from build123d import *

# Parameters (mm, degrees)
SKETCH1_R               = 2.2500000000000004
BOSS_EXTRUDE1_DEPTH     = 14
BOSS_EXTRUDE2_DEPTH     = 30
SKETCH3_R               = 7
CUT_EXTRUDE1_DEPTH      = 15
FILLET1_R               = 5
RIB1_REACH              = 65.484
SKETCH4_WALL_W          = 136.0395678423848
SKETCH4_WALL_H          = 4
FILLET2_R               = 5
BOSS_EXTRUDE3_START     = -6
SKETCH6_W               = 50
SKETCH6_H               = 20.33166445293904
BOSS_EXTRUDE3_DEPTH     = 5
CUT_EXTRUDE2_REACH      = 73.338
SKETCH7_R               = 8.250000000000005
SKETCH7_R_2             = 8.25
FILLET3_R               = 5
FILLET4_R               = 5
RIB2_REACH              = 68.324
SKETCH8_WALL_W          = 155.84718590256796
SKETCH8_WALL_H          = 4
FILLET5_R               = 3
CUT_EXTRUDE3_DEPTH      = 20
FILLET6_R               = 2
CUT_EXTRUDE4_REACH      = 93.033
CUT_EXTRUDE4_END_RADIUS = 7
SKETCH10_R              = 3.5000000000000004


with BuildPart() as part:
    # Sketch1 → Boss-Extrude1 (new body)
    with BuildSketch(Plane.XY):
        with BuildLine():
            Line((9.2e-16, 7.5), (-14.999999999999998, 7.500000000000002))
            Line((-14.999999999999998, 7.500000000000002), (-14.999999999999998, -7.500000000000002))
            Line((-14.999999999999998, -7.500000000000002), (9.2e-16, -7.5))
            ThreePointArc((9.2e-16, -7.5), (7.5, 0), (9.2e-16, 7.5))
        make_face()
        Circle(SKETCH1_R, mode=Mode.SUBTRACT)
    extrude(amount=BOSS_EXTRUDE1_DEPTH)

    # Sketch2 → Boss-Extrude2 (add)
    with BuildSketch(Plane.ZY.offset(14.999999999999998)):
        Polygon((-28.999999999999993, -7.500000000000002), (43, -7.500000000000002), (42.99999999999999, 12.499999999999998), (-28.99999999999999, 12.499999999999998), align=None)
    extrude(amount=BOSS_EXTRUDE2_DEPTH)

    # Sketch3 → Cut-Extrude1 (cut)
    with BuildSketch(Plane.ZY.offset(45)):
        with Locations((28.999999999999996, 2.499999999999998)):
            Circle(SKETCH3_R)
        with Locations((-15, 2.499999999999998)):
            Circle(SKETCH3_R)
    extrude(amount=-CUT_EXTRUDE1_DEPTH, mode=Mode.SUBTRACT)

    # Fillet1
    fillet1_edges = [part.edges().sort_by_distance(p)[0] for p in [
        (-30, 12.499999999999998, -28.99999999999999),
        (-30, -7.500000000000002, -28.999999999999993),
        (-30, -7.500000000000002, 43),
        (-30, 12.499999999999998, 42.99999999999999),
    ]]
    fillet(fillet1_edges, radius=FILLET1_R)

    # Sketch4 wall → Rib1 (add, up to next)
    with BuildSketch(Plane(origin=(-12.5, 10, 14), x_dir=(0.707106781187, -0.707106781187, 0), z_dir=(0.707106781187, 0.707106781187, 0)), mode=Mode.PRIVATE) as rib1_sk1:
        with Locations((0, 2)):
            Rectangle(SKETCH4_WALL_W, SKETCH4_WALL_H)
    rib1_tool1 = extrude(rib1_sk1.sketch, amount=-RIB1_REACH, mode=Mode.PRIVATE) - part.part
    rib1 = rib1_tool1.solids().sort_by_distance((-12.5, 10, 14))[0]
    add(rib1)

    # Mirror1: Rib1 across plane
    add(rib1.mirror(Plane.XY.offset(7)))

    # Fillet2
    fillet2_edges = [part.edges().sort_by_distance(p)[0] for p in [
        (-10.000000000000002, 7.500000000000001, 2),
        (-10.000000000000002, 7.500000000000001, 12),
    ]]
    fillet(fillet2_edges, radius=FILLET2_R)

    # Sketch6 → Boss-Extrude3 (add)
    with BuildSketch(Plane.ZY.offset(45).offset(BOSS_EXTRUDE3_START)):
        with Locations((7.000000000000005, 22.665832226469526)):
            Rectangle(SKETCH6_W, SKETCH6_H)
    extrude(amount=-BOSS_EXTRUDE3_DEPTH)

    # Sketch7 → Cut-Extrude2 (cut, up to next)
    with BuildSketch(Plane.ZY.offset(39), mode=Mode.PRIVATE) as cut_extrude2_sk1:
        with Locations((-5.999999999999993, 22.665832226469526)):
            Circle(SKETCH7_R)
    cut_extrude2_tool1 = extrude(cut_extrude2_sk1.sketch, amount=-CUT_EXTRUDE2_REACH, mode=Mode.PRIVATE) & part.part
    # Sketch7 → Cut-Extrude2 (cut, up to next)
    with BuildSketch(Plane.ZY.offset(39), mode=Mode.PRIVATE) as cut_extrude2_sk2:
        with Locations((20.000000000000007, 22.665832226469526)):
            Circle(SKETCH7_R_2)
    cut_extrude2_tool2 = extrude(cut_extrude2_sk2.sketch, amount=-CUT_EXTRUDE2_REACH, mode=Mode.PRIVATE) & part.part
    add(cut_extrude2_tool1.solids().sort_by_distance((-39, 22.665832, -6))[0], mode=Mode.SUBTRACT)
    add(cut_extrude2_tool2.solids().sort_by_distance((-39, 22.665832, 20))[0], mode=Mode.SUBTRACT)

    # Fillet3
    fillet3_edges = [part.edges().sort_by_distance(p)[0] for p in [
        (-36.5, 12.500000000000004, -17.999999999999996),
        (-36.5, 12.500000000000004, 32.00000000000001),
    ]]
    fillet(fillet3_edges, radius=FILLET3_R)

    # Fillet4
    fillet4_edges = [part.edges().sort_by_distance(p)[0] for p in [
        (-36.5, 32.831664452939044, -17.999999999999996),
        (-36.5, 32.831664452939044, 32.00000000000001),
    ]]
    fillet(fillet4_edges, radius=FILLET4_R)

    # Sketch8 wall → Rib2 (add, up to next)
    with BuildSketch(Plane(origin=(-42, 22.665832227, 7), x_dir=(-0.283038838463, -0.959108448467, 0), z_dir=(0.959108448467, -0.283038838463, 0)), mode=Mode.PRIVATE) as rib2_sk1:
        Rectangle(SKETCH8_WALL_W, SKETCH8_WALL_H)
    rib2_tool1 = extrude(rib2_sk1.sketch, amount=RIB2_REACH, mode=Mode.PRIVATE) - part.part
    add(rib2_tool1.solids().sort_by_distance((-42, 22.665832227, 7))[0])

    # Fillet5
    fillet5_edges = [part.edges().sort_by_distance(p)[0] for p in [
        (-42, 12.5, 9),
        (-42, 12.5, 5),
    ]]
    fillet(fillet5_edges, radius=FILLET5_R)

    # Sketch9 → Cut-Extrude3 (cut)
    with BuildSketch(Plane.ZY.offset(45)):
        with BuildLine():
            Line((-10.499999999999998, 10.499999999999998), (24.500000000000004, 10.499999999999998))
            ThreePointArc((24.500000000000004, 10.499999999999998), (16.500000000000004, 2.4999999999999996), (24.500000000000004, -5.500000000000002))
            Line((24.500000000000004, -5.500000000000002), (-10.499999999999998, -5.500000000000002))
            ThreePointArc((-10.499999999999998, -5.500000000000002), (-2.4999999999999982, 2.4999999999999987), (-10.499999999999998, 10.499999999999998))
        make_face()
    extrude(amount=-CUT_EXTRUDE3_DEPTH, mode=Mode.SUBTRACT)

    # Fillet6
    fillet6_edges = [part.edges().sort_by_distance(p)[0] for p in [
        (-35, -5.500000000000002, -10.499999999999998),
        (-35, 10.5, -10.499999999999996),
        (-35, 10.499999999999998, 24.500000000000004),
        (-35, -5.500000000000002, 24.500000000000004),
    ]]
    fillet(fillet6_edges, radius=FILLET6_R - 0.0001)  # a hair under: the kernel refuses the full size

    # Cut-Extrude4: up to this cylinder (the profile starts outside it)
    cut_extrude4_end = Plane(origin=(-37.5, 2.499999999999998, -15), z_dir=(-1, 0, 0)) * Cylinder(CUT_EXTRUDE4_END_RADIUS, 201.066, mode=Mode.PRIVATE)
    # Sketch10 → Cut-Extrude4 (cut, up to the surface)
    with BuildSketch(Plane(origin=(0, 5.03e-15, -28.999999999999993), x_dir=(-1, 0, 0), z_dir=(0, 1.7e-16, -1)), mode=Mode.PRIVATE) as cut_extrude4_sk1:
        with Locations(Location((37.5, 2.499999999999993, 0), (0, 0, 90))):
            Circle(SKETCH10_R)
    cut_extrude4_tool1 = extrude(cut_extrude4_sk1.sketch, amount=-CUT_EXTRUDE4_REACH, mode=Mode.PRIVATE) - cut_extrude4_end
    cut_extrude4 = cut_extrude4_tool1.solids().sort_by_distance((-37.5, 2.5, -29))[0]
    add(cut_extrude4, mode=Mode.SUBTRACT)

    # Mirror2: Cut-Extrude4 across plane
    add(cut_extrude4.mirror(Plane.XY.offset(7)), mode=Mode.SUBTRACT)


solid = part.part
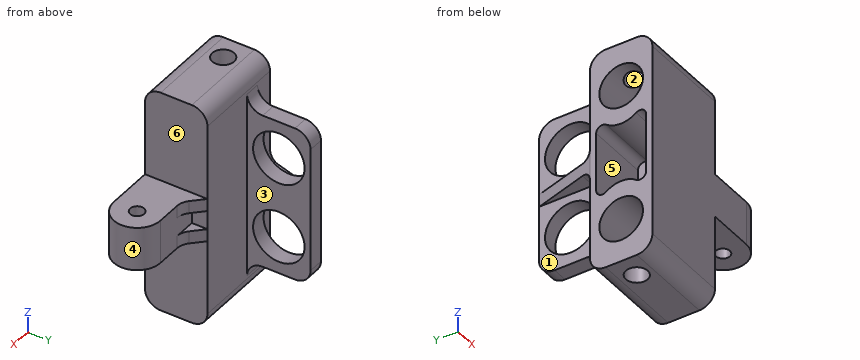
The listing builds one solid part. Answer for the finished solid, in the listing's coordinates (mm). Face numbers are marked on the shaded views. A direction names the side the tool comes from. Coordinates: 2 decimals unless noted, no trailing zeros. Order: outer loops, then holes, each group sorted by start corner. A loop starts at its lowest first (then second) coordinate and runs counter-clockwise, first axis right, second up.
Q1. A cutting plane is placed at B-B, the plane z = 7. Write down the section's boundary in (x, y), and give its area (3 significant figures).
Q2. For a pull along Y with two mould halves and no side action, classify the marked faces 4, 5 and 6 as pulls with the +Y half, pulls with the -Y half, needs draft (parallel to the pull), parting line crosses it, or undercut.
Q3. A cutting plane is placed at C-C, the plane y = 29.5. Write down the section's boundary in (x, z), and give its area (3 significant figures).
Q4. A cutting plane is placed at A-A, the plane z = -6. Write down the section's boundary in (x, y).
Q5. A cutting plane is placed at D-D, the plane z = -20. Write down the section's boundary in (x, y), and give its area (3 significant figures).
Q6. Given P1, Ø1.5, axis at x = -19, z = 29, coming from the +Y side; P2, Ø10, axis at y = 25.5, z = 27.5, coming from the -X side; P3, Ø10, axis at y = 22.67, z = 20, coming from the -X side; P4, Ø12.5, axis at y = 2.5, z = 29, coming from the +X side, each flat-ended and moving along its own axis, determine where each tip first touches the part or whether it passes through.
Q7. Which of the six approach directions +Z, -Z, +X, -X, +Y, -Y give full straight-line access (tool end or side, diameter ignored) to the marked faces 1, 2 and 3?
Q8. Consider line 1 (Y direction, x = -35, z = 9); line 2 (Y direction, x = -36, z = -6); line 3 (Z direction, x = -33, y = -3). Determine where each line is inside the solid, lowest interval first.
Answers follow:
1. outline: (-45, -7.5) - (0, -7.5) arc R7.5 ccw to (0, 7.5) - (-15, 7.5) - (-15, 12.5) - (-34, 12.5) - (-34, 32.83) - (-39, 32.83) - (-45, 12.5) - (-45, 10.5) - (-25, 10.5) - (-25, -5.5) - (-45, -5.5) - close; hole circle Ø4.5 at (0, 0)
1. area: 740 mm2
2. face 4: parting line crosses it
2. face 5: undercut
2. face 6: needs draft
3. outline: (-39.98, 5) - (-39, 5) - (-39, -1.38) - (-34, -1.38) - (-34, 15.38) - (-39, 15.38) - (-39, 9) - (-39.98, 9) - close; (-39, -17.71) - (-34, -17.71) - (-34, -10.62) - (-39, -10.62) - close; (-39, 24.62) - (-34, 24.62) - (-34, 31.71) - (-39, 31.71) - close
3. area: 159 mm2
4. outline: (-45, -7.5) - (-15, -7.5) - (-15, 12.5) - (-34, 12.5) - (-34, 14.42) - (-39, 14.42) - (-39, 12.5) - (-45, 12.5) - close; (-39, 30.92) - (-34, 30.92) - (-34, 32.83) - (-39, 32.83) - close
5. outline: (-45, -7.5) - (-15, -7.5) - (-15, 12.5) - (-34, 12.5) - (-34, 13.5) - (-39, 13.5) - (-39, 12.5) - (-45, 12.5) - (-45, 7.4) - (-30, 7.4) - (-30, -2.4) - (-45, -2.4) - close
5. area: 458 mm2
6. P1: stops at y = 12.5
6. P2: stops at x = -39
6. P3: passes through
6. P4: stops at x = -15
7. face 1: -Z, -X, +Y
7. face 2: +Z
7. face 3: +Z, -Z, +X, +Y
8. line 1: y = -7.5 to -5.5, 10.5 to 32.83
8. line 2: y = -7.5 to 14.42, 30.92 to 32.83
8. line 3: z = -28.97 to -19.33, -10.67 to -4.44, 18.44 to 24.67, 33.33 to 42.97
